```python
from build123d import *

# Parameters (mm, degrees)
SKETCH_1_W               = 60
SKETCH_1_H               = 106
EXTRUDE_1_DEPTH          = 15
CUT_EXTRUDE_1_DEPTH      = 10
CUT_EXTRUDE_2_DEPTH      = 63.721607122
CUT_EXTRUDE_2_DEPTH_BACK = 63.721607122
SKETCH_3_R               = 2.1


with BuildPart() as part:
    # 草图1 → 凸台-拉伸1 (new body)
    with BuildSketch(Plane(origin=(0, 0, 0), x_dir=(1, 0, 0), z_dir=(0, 1, 0))):
        Rectangle(SKETCH_1_W, SKETCH_1_H)
    extrude(amount=EXTRUDE_1_DEPTH)

    # 草图2 → 切除-拉伸1 (cut)
    with BuildSketch(Plane.XZ):
        Polygon((-32.957810335, 43), (38.640191428, 43), (38.640191428, 38), (-35.799000882, 38), align=None)
        Polygon((38.640191428, -38), (-35.799000882, -38), (-32.957810335, -43), (38.640191428, -43), align=None)
    extrude(amount=-CUT_EXTRUDE_1_DEPTH, mode=Mode.SUBTRACT)

    # 草图3 → 切除-拉伸2 (cut, two sides: drawn at the far end of the back side and taken through both)
    with BuildSketch(Plane(origin=(0, 15, 0), x_dir=(1, 0, 0), z_dir=(0, 1, 0)).offset(-CUT_EXTRUDE_2_DEPTH_BACK)):
        with Locations(Location((0, 0, 0), (0, 0, 270))):
            Circle(SKETCH_3_R)
    extrude(amount=CUT_EXTRUDE_2_DEPTH + CUT_EXTRUDE_2_DEPTH_BACK, mode=Mode.SUBTRACT)


solid = part.part
```
Build history of the part. All positions in model axes, mm. A direction names the side the tool comes from. Give positions to 0.01 mm unless a question says otherwise; leave off trailing zeros. Loops run counter-clockwise (first coordinate to the right, second up) from the corner with the lowest first, then second, coordinate; pieces in that order, holes last.
Item 1: Slice it at C-C, the plane z = 0. List the corners of the cut face in (x, y).
Answers follow:
outline: (-30, 0) - (-2.1, 0) - (-2.1, 15) - (-30, 15) - close; (2.1, 0) - (30, 0) - (30, 15) - (2.1, 15) - close
Item 2: Pull direction Z, two halves, no side cores. Call faces 3 (the face through (-30, 7, 1)), 4 (the face through (0, 7, -53)), 5 (the face through (0, 5, 38)): released by +Z, released by -Z, zero draft, split by the parting line, or undercut.
Answers follow:
face 3: zero draft
face 4: released by -Z
face 5: undercut
Item 3: Slice it at A-A, the plane x = 0. List the corners of the cut face in (y, z).
Answers follow:
outline: (0, -53) - (15, -53) - (15, -2.1) - (0, -2.1) - (0, -38) - (10, -38) - (10, -43) - (0, -43) - close; (0, 2.1) - (15, 2.1) - (15, 53) - (0, 53) - (0, 43) - (10, 43) - (10, 38) - (0, 38) - close
Item 4: Slice it at B-B, the plane y = 7.75. List the corners of the cut face in (x, z), and give its area (3 significant figures).
Answers follow:
outline: (-30, -53) - (30, -53) - (30, -43) - (-30, -43) - close; (-30, -38) - (30, -38) - (30, 38) - (-30, 38) - close; (-30, 43) - (30, 43) - (30, 53) - (-30, 53) - close; hole circle Ø4.2 at (0, 0)
area: 5,750 mm2
Item 5: Slice it at D-D, the plane x = -14. List the corners of the cut face in (y, z), and give its area (3 significant figures).
Answers follow:
outline: (0, -53) - (15, -53) - (15, 53) - (0, 53) - (0, 43) - (10, 43) - (10, 38) - (0, 38) - (0, -38) - (10, -38) - (10, -43) - (0, -43) - close
area: 1,490 mm2
Item 6: Flat gauge pins, fed straight in: pin 1 (2.5 mm diameter, centred on x = 5, z = 39.5, fed in from -Y); pin 2 (2.5 mm diameter, centred on x = 0, z = 0, fed in from +Y). Where does each tip first touch, or does it go through?
Answers follow:
pin 1: stops at y = 10
pin 2: passes through
Item 7: Which spindle directions (+Z, -Z, +X, -X, +Y, -Y) get a long thin tool onto all of the face, cutting with end or side? Do faces 1 (the face through (-7, 0, -1)), 2 (the face through (0, 5, -43)). Say none if no direction does.
Answers follow:
face 1: +Z, -Z, +X, -X, -Y
face 2: +X, -X, -Y
Item 8: Drill centre lines: line 1 (Z direction, x = -13.5, y = 2.25); line 2 (Z direction, x = 0, y = 7.25); line 3 (Z direction, x = 0, y = 11.5). Where is each one in solid material? Low to high.
Answers follow:
line 1: z = -53 to -43, -38 to 38, 43 to 53
line 2: z = -53 to -43, -38 to -2.1, 2.1 to 38, 43 to 53
line 3: z = -53 to -2.1, 2.1 to 53
